```python
from build123d import *

# Parameters (mm, degrees)
BOSS_EXTRUDE1_DEPTH     = 160
SKETCH3_R               = 1.5
CUT_EXTRUDE1_DEPTH      = 40.389262615
SKETCH4_R               = 4
CUT_EXTRUDE2_DEPTH      = 8
CUT_EXTRUDE3_DEPTH      = 19.147013842
CUT_EXTRUDE3_DEPTH_BACK = 31.333948183
SKETCH6_W               = 4
SKETCH6_H               = 14.600219614
CUT_EXTRUDE4_DEPTH      = 1
CUT_EXTRUDE4_DEPTH_BACK = 161


with BuildPart() as part:
    # Sketch1 → Boss-Extrude1 (new body)
    with BuildSketch(Plane.XY):
        Polygon((0, 0), (-78.530174676, -15.26471963), (-95.10565163, -30.901699437), align=None)
    extrude(amount=BOSS_EXTRUDE1_DEPTH)

    # Sketch3 → Cut-Extrude1 (cut, through all)
    with BuildSketch(Plane(origin=(-3.090169944, 9.510565163, 0), x_dir=(0.951056516, 0.309016994, 0), z_dir=(-0.309016994, 0.951056516, 0))):
        with Locations((-89.701846066, -20)):
            Circle(SKETCH3_R)
        with Locations((-89.701846066, -80)):
            Circle(SKETCH3_R)
        with Locations((-89.701846066, -140)):
            Circle(SKETCH3_R)
    extrude(amount=-CUT_EXTRUDE1_DEPTH, mode=Mode.SUBTRACT)

    # Sketch4 → Cut-Extrude2 (cut)
    with BuildSketch(Plane(origin=(-3.090169944, 9.510565163, 0), x_dir=(0.951056516, 0.309016994, 0), z_dir=(-0.309016994, 0.951056516, 0))):
        with Locations((-89.701846066, -20)):
            Circle(SKETCH4_R)
        with Locations((-89.701846066, -80)):
            Circle(SKETCH4_R)
        with Locations((-89.701846066, -140)):
            Circle(SKETCH4_R)
    extrude(amount=-CUT_EXTRUDE2_DEPTH, mode=Mode.SUBTRACT)

    # Sketch5 → Cut-Extrude3 (cut, two sides)
    with BuildSketch(Plane(origin=(-0.600388906, -0.116703781, 0), x_dir=(0.981627183, 0.190808995, 0), z_dir=(-0.190808995, 0.981627183, 0))) as cut_extrude3_sk:
        with BuildLine():
            Line((-49.109208006, -123.6), (-79.388373798, -123.6))
            ThreePointArc((-79.388373798, -123.6), (-82.988373798, -120), (-79.388373798, -116.4))
            Line((-79.388373798, -116.4), (-49.109208006, -116.4))
            ThreePointArc((-49.109208006, -116.4), (-45.509208006, -120), (-49.109208006, -123.6))
        make_face()
        with BuildLine():
            Line((-49.109208006, -83.6), (-79.388373798, -83.6))
            ThreePointArc((-79.388373798, -83.6), (-82.988373798, -80), (-79.388373798, -76.4))
            Line((-79.388373798, -76.4), (-49.109208006, -76.4))
            ThreePointArc((-49.109208006, -76.4), (-45.509208006, -80), (-49.109208006, -83.6))
        make_face()
        with BuildLine():
            Line((-49.109208006, -43.6), (-79.388373798, -43.6))
            ThreePointArc((-79.388373798, -43.6), (-82.988373798, -40), (-79.388373798, -36.4))
            Line((-79.388373798, -36.4), (-49.109208006, -36.4))
            ThreePointArc((-49.109208006, -36.4), (-45.509208006, -40), (-49.109208006, -43.6))
        make_face()
    extrude(amount=CUT_EXTRUDE3_DEPTH, mode=Mode.SUBTRACT)
    extrude(cut_extrude3_sk.sketch, amount=-CUT_EXTRUDE3_DEPTH_BACK, mode=Mode.SUBTRACT)

    # Sketch6 → Cut-Extrude4 (cut, two sides)
    with BuildSketch(Plane.XY.offset(160)) as cut_extrude4_sk:
        Polygon((-15, 4.492478665), (-15, -6.969839796), (0, -6.969839796), (0, 6.969839796), align=None)
        with Locations((-93.10565163, -29.084878329)):
            Rectangle(SKETCH6_W, SKETCH6_H)
    extrude(amount=CUT_EXTRUDE4_DEPTH, mode=Mode.SUBTRACT)
    extrude(cut_extrude4_sk.sketch, amount=-CUT_EXTRUDE4_DEPTH_BACK, mode=Mode.SUBTRACT)


solid = part.part
```
Check sheet for the modelled part. Datum: model origin and axes. Units: mm. A direction names the side the tool comes from. Round coordinates to 2 decimals unless told otherwise and drop trailing zeros. Write each loop counter-clockwise with the first axis right and the second up, starting at its lowest first coordinate (ties: lowest second). Pieces come first, ordered by that corner, then holes. Notation, with made-up numbers: (33, -18) -> (57, -18) arc R11 ccw to (57, -12) -> close; hole circle Ø6 at (-19.5, -18.5). An arc over 180 degrees is marked (long way). One line per question, with ' | ' between items. Start each with the question number.
1. Set-up check for faces 4 (the face through (-85.983, -25.835, 141.722)), 5 (the face through (-44.7, -11.75, 119.92)): record each of +Z, -Z, +X, -X, +Y, -Y from which the full face is reachable in a straight line by a thin tool's end or side.
2. Depth check by flat-ended pin: pin 1 (6 mm diameter, centred on y = -23, z = 134, fed in from -X); pin 2 (6 mm diameter, centred on x = -35.5, z = 127, fed in from +Y); pin 3 (10 mm diameter, centred on x = -55, z = 143.5, fed in from +Y). Enter the tip coordinate at first touch or a pass-through.
3. Scan lines: line 1 along Z through (x, y) = (-62.5, -14.75); line 2 along Y through (x, z) = (-21, 96); line 3 along Y through (x, z) = (-31, 32). Record each from-to range of solid material in increasing order. Write a range as from..to.
4. Sectioned sample at A-A, the plane x = -66.5. Record the cut outline in (y, z).
5. Sectioned sample at B-B, the plane z = 69. Record the cut outline in (x, y).
6. Sectioned sample at D-D, the plane x = -39. Record the cut outline in (y, z), then the cut area to 3 significant figures.
7. Release check for a two-part mould opening along Z. For faces 1 (the face through (-59, -15, 160)), 2 (the face through (-83.333, -19.795, 78.88)), 3 (the face through (-84.858, -26.506, 78.735)) record: +Z half, -Z half, draft (parallel to the pull), parting line (faces both ways), or undercut.
8. Sectioned sample at C-C, the plane y = -17.25. Count the separate pieces of the cut face and the enclosed holes in it, then the cut area to 3 significant figures.
Taken from the geometry:
1) face 4: none | face 5: -X, -Y
2) pin 1: stops at x = -89.91 | pin 2: stops at y = -6.32 | pin 3: stops at y = -9.72
3) line 1: z = 0..36.4, 43.6..76.4, 83.6..116.4, 123.6..160 | line 2: y = -6.82..-4.08 | line 3: y = -10.07..-6.03
4) outline: (-21.61, 0) -> (-12.93, 0) -> (-12.93, 36.4) -> (-21.61, 36.4) -> close; (-21.61, 43.6) -> (-12.93, 43.6) -> (-12.93, 76.4) -> (-21.61, 76.4) -> close; (-21.61, 83.6) -> (-12.93, 83.6) -> (-12.93, 116.4) -> (-21.61, 116.4) -> close; (-21.61, 123.6) -> (-12.93, 123.6) -> (-12.93, 160) -> (-21.61, 160) -> close
5) outline: (-91.11, -29.6) -> (-15, -4.87) -> (-15, -2.92) -> (-78.53, -15.26) -> (-91.11, -27.13) -> close
6) outline: (-12.67, 0) -> (-7.58, 0) -> (-7.58, 160) -> (-12.67, 160) -> close | area: 815 mm^2
7) face 1: +Z half | face 2: draft | face 3: undercut
8) separate pieces: 4 | enclosed holes: 0 | area: 3,820 mm^2
